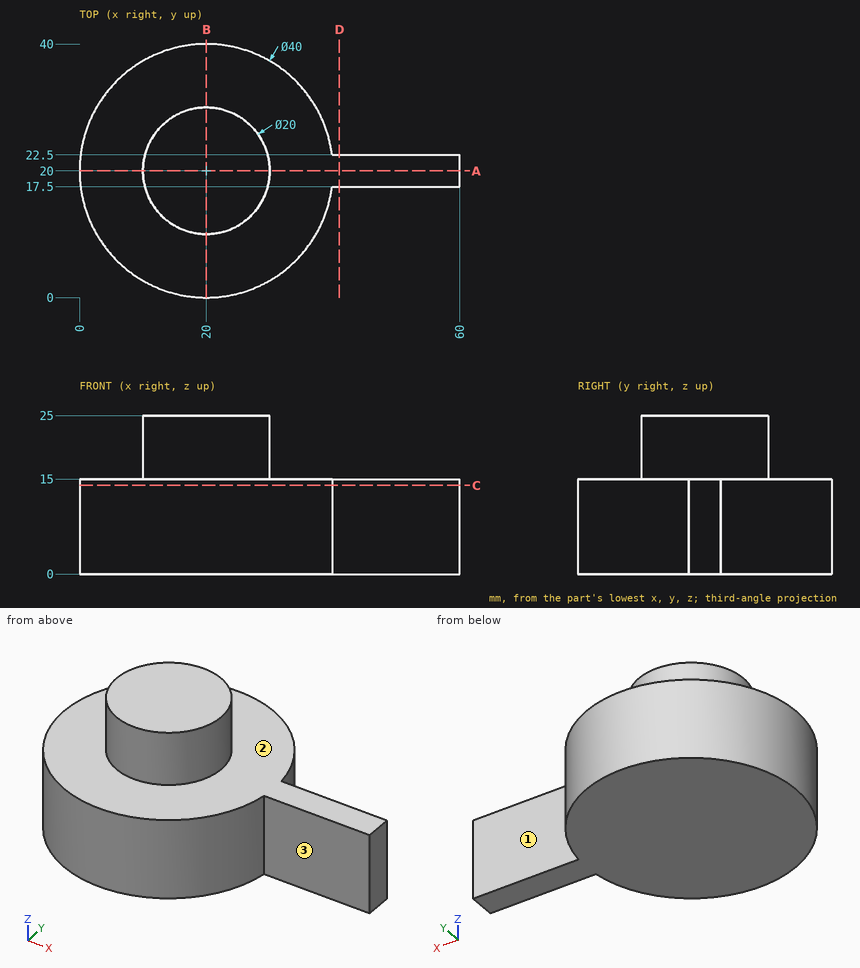
Source: three-view drawing plus pictorial views. Frame: mm from the lowest corner of the part. A direction names the side the tool comes from. Round coordinates to 2 decimals unless told otherwise and drop trailing zeros. Write each loop counter-clockwise with the first axis right and the second up, starting at its lowest first coordinate (ties: lowest second). Pieces come first, ordered by that corner, then holes. Notation, with made-up numbers: M 76,-4 L 119,-4 A35 cw 119,34 Z; hole C -21,-39.5 d5. An arc over 180 degrees is marked long. One line per item, written item: value. Start each with the question number.
Item 1: Ray query, L1, parallel to Z at x = 21, y = 31; L2, parallel to Y at x = 45, z = 5; L3, parallel to X at y = 19.5, z = 16.25. Return the intervals inside material, ascending. Write a range as from..to.
Item 2: Section query A-A (y = 20). Return the cut outline in (x, z).
Item 3: Set-up query: the marked faces 1, 2 and 3. Return all of +Z, -Z, +X, -X, +Y, -Y with unobstructed straight access to the full face (end or side cutting, diameter ignored); none if empty.
Item 4: Section query D-D (x = 41). Return the cut outline in (y, z), plus the area to 3 significant figures.
Item 5: Pin query (flat end, axial travel): pin 1 (1.5 mm diameter, centred on x = 11.5, z = 20.5, fed in from -Y); pin 2 (10 mm diameter, centred on y = 31, z = 8, fed in from -X); pin 3 (8 mm diameter, centred on y = 28, z = 11.5, fed in from -X). Return the tip coordinate at first contact, or that it passes through.
Item 6: Section query C-C (z = 14). Return the cut outline in (x, y).
Item 7: Section query B-B (x = 20). Return the cut outline in (y, z).
Result set:
1. L1: z = 0..15
1. L2: y = 17.5..22.5
1. L3: x = 10.01..29.99
2. outline: M 0,0 L 60,0 L 60,15 L 30,15 L 30,25 L 10,25 L 10,15 L 0,15 Z
3. face 1: +Z, -Z, +X, +Y
3. face 2: +Z
3. face 3: +Z, -Z, +X, -Y
4. outline: M 17.5,0 L 22.5,0 L 22.5,15 L 17.5,15 Z
4. area: 75.0 mm²
5. pin 1: stops at y = 13.68
5. pin 2: stops at x = 0.92
5. pin 3: stops at x = 0.4
6. outline: M 39.84,17.5 L 60,17.5 L 60,22.5 L 39.84,22.5 A20 ccw long Z
7. outline: M 0,0 L 40,0 L 40,15 L 30,15 L 30,25 L 10,25 L 10,15 L 0,15 Z
